```python
from build123d import *

# Parameters (mm, degrees)
F0_R     = 2.5
F1_DEPTH = 2.5
F0_R_2   = 1.3
F2_DEPTH = 7.5
F3_DEPTH = 90
F4_DEPTH = 1.3


with BuildPart() as f1:
    # F0 (on Top) → F1 (new body)
    with BuildSketch(Plane.XY):
        with BuildLine():
            Line((8.9, 21.9654273803), (8.9, -21.9654273803))
            ThreePointArc((8.9, -21.9654273803), (23.7, 0), (8.9, 21.9654273803))
        make_face()
        with BuildLine():
            ThreePointArc((10.2, 19.9429185427), (22.4, 0), (10.2, -19.9429185427))
            Line((10.2, -19.9429185427), (10.2, 19.9429185427))
        make_face(mode=Mode.SUBTRACT)
        with BuildLine():
            Line((10.2, 19.9429185427), (10.2, -19.9429185427))
            ThreePointArc((10.2, -19.9429185427), (22.4, 0), (10.2, 19.9429185427))
        make_face()
        with Locations((13.9515874907, 11.5695847198)):
            Circle(F0_R, mode=Mode.SUBTRACT)
    extrude(amount=F1_DEPTH)

    # F0 (on Top) → F2 (join)
    with BuildSketch(Plane.XY):
        with Locations((13.9515874907, 11.5695847198)):
            Circle(F0_R)
        with Locations((13.9515874907, 11.5695847198)):
            Circle(F0_R_2, mode=Mode.SUBTRACT)
    extrude(amount=F2_DEPTH)

    # F3 (add): a face of the model
    f3_faces = [f1.faces().sort_by_distance(p)[0] for p in [
        (11.5222981689, 11.5695847198, 7.5),
    ]]
    extrude(f3_faces, amount=-F3_DEPTH)

    # F0 (on Top) → F4 (cut)
    with BuildSketch(Plane.XY):
        with BuildLine():
            Line((8.9, 21.9654273803), (8.9, -21.9654273803))
            ThreePointArc((8.9, -21.9654273803), (23.7, 0), (8.9, 21.9654273803))
        make_face()
        with BuildLine():
            ThreePointArc((10.2, 19.9429185427), (22.4, 0), (10.2, -19.9429185427))
            Line((10.2, -19.9429185427), (10.2, 19.9429185427))
        make_face(mode=Mode.SUBTRACT)
    extrude(amount=F4_DEPTH, mode=Mode.SUBTRACT)


solid = f1.part
```
Could you check a few things on this model? Use its own coordinates, in mm. A direction names the side the tool comes from. Round coordinates to 2 decimals unless told otherwise and drop trailing zeros. Loops run counter-clockwise (first coordinate to the right, second up) from the corner with the lowest first, then second, coordinate; pieces in that order, holes last. Notation, with made-up numbers: M 30,46.25 L 36,46.25 A21 cw 36,70.25 Z; hole C 57,71.25 d3. An arc over 180 degrees is marked long. Answer as CSV lines item,"result".
1) Imagine slicing it at B-B on x = 18. List the corners of the cut face in (y, z) for me, and give its area (3 significant figures).
From the geometry:
outline,"M -15.42,1.3 L -13.33,1.3 L -13.33,0 L 13.33,0 L 13.33,1.3 L 15.42,1.3 L 15.42,2.5 L -15.42,2.5 Z"
area,"71.7 mm^2"
2) Imagine slicing it at A-A on y = 6. List the corners of the cut face in (x, z) for me, and give its area (3 significant figures).
From the geometry:
outline,"M 8.9,1.3 L 10.2,1.3 L 10.2,0 L 21.58,0 L 21.58,1.3 L 22.93,1.3 L 22.93,2.5 L 8.9,2.5 Z"
area,"31.6 mm^2"
3) Which directions (+Z, -Z, +X, -X, +Y, -Y) give clear straight access to the entire face, cutting with the end or side of a thin tool? Please do faces 1 (the cylindrical face through (22.397, 0.344, 0.641)), 2 (the flat face through (10, 0, 1.3)), 3 (the cylindrical face through (11.454, 11.68, 4.965)).
From the geometry:
face 1,"-Z, +X"
face 2,"-Z"
face 3,"+Z"
4) For pin 1 Ø8 at (x, z) = (16.5, -16) entering from +Y; pin 2 Ø4 at (x, y) = (21.5, 7) entering from +Z; pin 3 Ø8 at (x, z) = (13, -41) entering from -Y; pin 4 Ø3 at (x, y) = (13.95, 11.57) entering from -Z, each with a flat end and sliding along its axis, tell me the tip position at first contact or that it passes through.
From the geometry:
pin 1,"y = 14.07"
pin 2,"z = 2.5"
pin 3,"y = 9.07"
pin 4,"z = -82.5"
5) Imagine slicing it at C-C on z = -37. List the corners of the cut face in (x, y) for me, and give its area (3 significant figures).
From the geometry:
outline,"C 13.95,11.57 d5; hole C 13.95,11.57 d2.6"
area,"14.3 mm^2"
6) If I drill on probe 1 along Z at (x, y) = (11.5, 5); probe 2 along Z at (x, y) = (22.5, -0.5); probe 3 along Y at (x, z) = (15, -12), over which ranges is the centre line in solid material (lowest first)?
From the geometry:
probe 1,"0 to 2.5"
probe 2,"1.3 to 2.5"
probe 3,"9.3 to 10.8, 12.34 to 13.84"
